from build123d import *

# Parameters (mm, degrees)
SKETCH1_R                    = 12.7
BOSS_EXTRUDE1_DEPTH          = 25.4
SKETCH2_R                    = 7.9375
CUT_EXTRUDE1_DEPTH           = 3.175
SKETCH12_R                   = 1.999996
BOSS_EXTRUDE3_DEPTH          = 12.7
F_1_8_0_125_DIAMETER_HOLE1_D = 3.175


with BuildPart() as part:
    # Sketch1 → Boss-Extrude1 (new body)
    with BuildSketch(Plane(origin=(0, 0, 0), x_dir=(1, 0, 0), z_dir=(0, 1, 0))):
        with Locations(Location((0, 0, 0), (0, 0, 270))):
            Circle(SKETCH1_R)
    extrude(amount=BOSS_EXTRUDE1_DEPTH)

    # Sketch2 → Cut-Extrude1 (cut)
    with BuildSketch(Plane(origin=(0, 0, 0), x_dir=(1, 0, 0), z_dir=(0, 1, 0))):
        with Locations(Location((0, 0, 0), (0, 0, 270))):
            Circle(SKETCH2_R)
    extrude(amount=CUT_EXTRUDE1_DEPTH, mode=Mode.SUBTRACT)

    # Sketch12 → Boss-Extrude3 (add)
    with BuildSketch(Plane(origin=(0, 25.4, 0), x_dir=(1, 0, 0), z_dir=(0, 1, 0))):
        with Locations(Location((0, 0, 0), (0, 0, 270))):
            Circle(SKETCH12_R)
    extrude(amount=BOSS_EXTRUDE3_DEPTH)

    # 1/8 (0.125) Diameter Hole1 (through all)
    with Locations(Plane(origin=(0, 3.175, 0), x_dir=(-1, 0, 0), z_dir=(0, -1, 0))):
        with Locations((0, 0)):
            Hole(F_1_8_0_125_DIAMETER_HOLE1_D / 2)


solid = part.part
The listing builds one solid part. Answer for the finished solid, in the listing's coordinates (mm). A direction names the side the tool comes from. Round coordinates to 2 decimals unless told otherwise and drop trailing zeros. Loops run counter-clockwise (first coordinate to the right, second up) from the corner with the lowest first, then second, coordinate; pieces in that order, holes last. Notation, with made-up numbers: M 53,-28.75 L 110,-28.75 A13 ccw 110,-7.75 Z; hole C 61.5,56 d1. An arc over 180 degrees is marked long. Write each question's results on one line, items separated by ' | '. Start each with the question number.
1) Each of these flat-tipped pins is pushed along its axis until it touches: pin 1 (2 mm diameter, centred on y = 24.5, z = 8, fed in from +X); pin 2 (1.5 mm diameter, centred on x = 3, y = 16, fed in from -Z); pin 3 (3 mm diameter, centred on y = 13, z = -4.5, fed in from -X). Where does it stop, or does it pass through?
2) Find section C-C on y = 22.5. Write down the section's boundary in (x, z) (1 decimal), plus the area to 3 significant figures.
3) Straight lines are drawn through the part: probe 1 along X at (y, z) = (1.1, 0); probe 2 along Y at (x, z) = (1, 7) (3 decimals); probe 3 along X at (y, z) = (27, 0.75). For each, find the intervals that lie inside material, in ascending order.
4) Determine the mould class of faces 3 (the flat face through (-8.3, 0, -0.2)), 4 (the cylindrical face through (-7.7, 12.5, -10.1)), 5 (the cylindrical face through (-0.34, 20.88, 1.55)) for opening direction Z: pulls with the +Z half, pulls with the -Z half, needs draft (parallel to the pull), parting line crosses it, or undercut.
5) Find section D-D on x = -3.75. Write down the section's boundary in (y, z) (3 decimals).
6) Find section B-B on z = 0. Write down the section's boundary in (x, y) (1 decimal), plus the area to 3 significant figures.
7) Find section A-A on x = 0. Write down the section's boundary in (y, z) (1 decimal).
8) Which of the six approach directions +Z, -Z, +X, -X, +Y, -Y give full straight-line access (tool end or side, diameter ignored) to faces 1 (the cylindrical face through (-1.2, 31.7, -1.6)), 2 (the cylindrical face through (-7.75, 1.57, -1.72))?
Final values:
1) pin 1: x = 10.6 | pin 2: z = -12.5 | pin 3: x = -12.34
2) outline: C 0,0 d25.4; hole C 0,0 d3.2 | area: 499 mm²
3) probe 1: -12.7 to -7.94, 7.94 to 12.7 | probe 2: 3.175 to 25.4 | probe 3: -1.85 to -1.4, 1.4 to 1.85
4) face 3: needs draft | face 4: parting line crosses it | face 5: undercut
5) outline: M 0,-12.134 L 25.4,-12.134 L 25.4,12.134 L 0,12.134 L 0,6.996 L 3.175,6.996 L 3.175,-6.996 L 0,-6.996 Z
6) outline: M -12.7,0 L -7.9,0 L -7.9,3.2 L -1.6,3.2 L -1.6,38.1 L -2,38.1 L -2,25.4 L -12.7,25.4 Z; M 1.6,3.2 L 7.9,3.2 L 7.9,0 L 12.7,0 L 12.7,25.4 L 2,25.4 L 2,38.1 L 1.6,38.1 Z | area: 535 mm²
7) outline: M 0,-12.7 L 25.4,-12.7 L 25.4,-2 L 38.1,-2 L 38.1,-1.6 L 3.2,-1.6 L 3.2,-7.9 L 0,-7.9 Z; M 0,7.9 L 3.2,7.9 L 3.2,1.6 L 38.1,1.6 L 38.1,2 L 25.4,2 L 25.4,12.7 L 0,12.7 Z
8) face 1: +Y | face 2: -Y
